Could you check a few things on this drawing? It's one solid part, dimensions in mm from its lowest x, y, z. A direction names the side the tool comes from. Give positions to 0.01 mm unless a question says otherwise; leave off trailing zeros. Loops run counter-clockwise (first coordinate to the right, second up) from the corner with the lowest first, then second, coordinate; pieces in that order, holes last. Notation, with made-up numbers: M 1,-22 L 33,-22 A28 cw 33,2 Z; hole C 3.25,61.25 d10. An arc over 180 degrees is marked long. Return JSON: item names as keys, results as strings. Group by question number.
1. If we section it at D-D (x = 43): Write out the boundary of the cut face in (y, z).
2. For the marked faces 1, 2, 3, 4 and 5, which set-ups out of +Z, -Z, +X, -X, +Y, -Y let a thin tool reach every point of the face, with its end or its side?
3. If we mould it in two halves opening along Z, with no side actions, what happens to the marked faces 6, 7 and 8? For each: +Z half, -Z half, draft (parallel to the pull), parting line (faces both ways), or undercut.
4. If we section it at B-B (x = 53.5): Write out the boundary of the cut face in (y, z), plus the area to 3 significant figures.
5. For pin 1 (3 mm diameter, centred on y = 22, z = 110.5, fed in from -X); pin 2 (6 mm diameter, centred on x = 12.5, y = 18, fed in from -Z); pin 3 (7.5 mm diameter, centred on y = 42, z = 13, fed in from +X); pin 4 (12 mm diameter, centred on x = 62.5, y = 21, fed in from +Z), each with a flat end and sliding along its axis, tell me the tip position at first contact or that it passes through.
6. If we section it at A-A (x = 26.5): Write out the boundary of the cut face in (y, z), plus the area to 3 significant figures.
7. Please list where these lines run through material, in increasing order: line 1 (X direction, y = 46.5, z = 64); line 2 (Z direction, x = 63, y = 29); line 3 (X direction, y = 31, z = 10).
8. If we section it at C-C (y = 27): Write out the boundary of the cut face in (x, z).
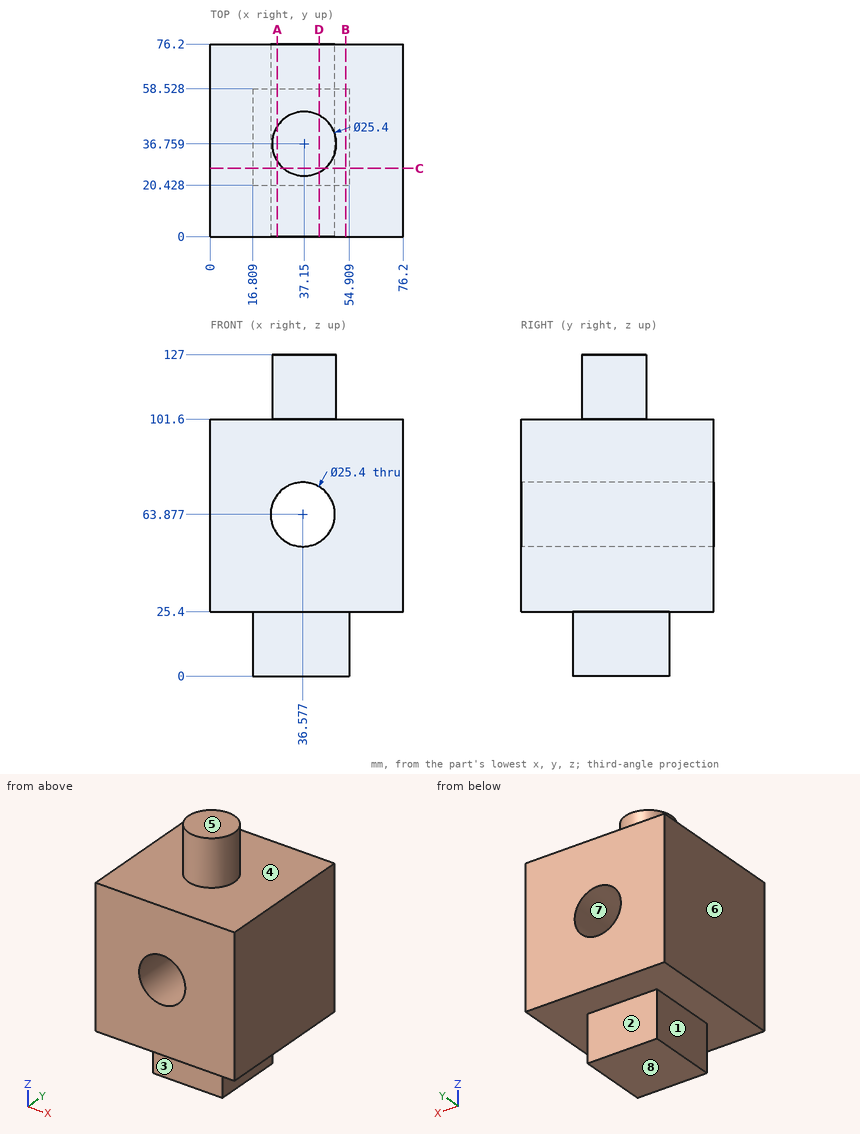
Answer:
{
 "1": {"outline": "M 0,25.4 L 20.43,25.4 L 20.43,0 L 58.53,0 L 58.53,25.4 L 76.2,25.4 L 76.2,52.92 L 0,52.92 Z; M 0,74.83 L 76.2,74.83 L 76.2,101.6 L 48.03,101.6 L 48.03,127 L 25.49,127 L 25.49,101.6 L 0,101.6 Z"},
 "2": {"face 1": "-Z, -X, +Y, -Y", "face 2": "-Z, +X, -X, +Y", "face 3": "-Z, +X, -X, -Y", "face 4": "+Z", "face 5": "+Z, +X, -X, +Y, -Y"},
 "3": {"face 6": "draft", "face 7": "undercut", "face 8": "-Z half"},
 "4": {"outline": "M 0,25.4 L 20.43,25.4 L 20.43,0 L 58.53,0 L 58.53,25.4 L 76.2,25.4 L 76.2,101.6 L 0,101.6 Z", "area": "6,770 mm²"},
 "5": {"pin 1": "passes through", "pin 2": "stops at z = 25.4", "pin 3": "stops at x = 54.91", "pin 4": "stops at z = 101.6"},
 "6": {"outline": "M 0,25.4 L 20.43,25.4 L 20.43,0 L 58.53,0 L 58.53,25.4 L 76.2,25.4 L 76.2,56.15 L 0,56.15 Z; M 0,71.61 L 76.2,71.61 L 76.2,101.6 L 43.68,101.6 L 43.68,127 L 29.84,127 L 29.84,101.6 L 0,101.6 Z", "area": "5,950 mm²"},
 "7": {"line 1": "x = 0 to 23.88, 49.28 to 76.2", "line 2": "z = 25.4 to 101.6", "line 3": "x = 16.81 to 54.91"},
 "8": {"outline": "M 0,25.4 L 16.81,25.4 L 16.81,0 L 54.91,0 L 54.91,25.4 L 76.2,25.4 L 76.2,101.6 L 45.28,101.6 L 45.28,127 L 29.02,127 L 29.02,101.6 L 0,101.6 Z; hole C 36.58,63.88 d25.4"}
}
